```python
from build123d import *

# Parameters (mm, degrees)
F0_R     = 28.575
F0_R_2   = 2.032
F1_DEPTH = 3.175
F2_R     = 13.97
F3_DEPTH = 6.35
F5_DEPTH = 9.525
F7_DEPTH = 9.525
F8_R     = 12.954
F8_R_2   = 1.8288
F9_DEPTH = 3.175


with BuildPart() as f1:
    # F0 (on Top) → F1 (new body)
    with BuildSketch(Plane.XY):
        Circle(F0_R)
        with Locations((-20.6222299276, -11.90625)):
            Circle(F0_R_2, mode=Mode.SUBTRACT)
        with Locations((0, -23.8125)):
            Circle(F0_R_2, mode=Mode.SUBTRACT)
        with Locations((20.6222299276, -11.90625)):
            Circle(F0_R_2, mode=Mode.SUBTRACT)
        with Locations((-20.6222299276, 11.90625)):
            Circle(F0_R_2, mode=Mode.SUBTRACT)
        with Locations((20.6222299276, 11.90625)):
            Circle(F0_R_2, mode=Mode.SUBTRACT)
        with Locations((0, 23.8125)):
            Circle(F0_R_2, mode=Mode.SUBTRACT)
    extrude(amount=F1_DEPTH)

    # F2 (on face) → F3 (join)
    with BuildSketch(Plane.XY.offset(3.175)):
        Circle(F2_R)
    extrude(amount=F3_DEPTH)

    # F4 (on face) → F5 (cut, through all)
    with BuildSketch(Plane(origin=(0, 0, 0), x_dir=(1, 0, 0), z_dir=(0, 0, -1))):
        with BuildLine():
            ThreePointArc((-1.987864432, 2.794), (-1.5718864244, -3.0474930793), (3.429, 0))
            ThreePointArc((3.429, 0), (3.0474930793, 1.5718864244), (1.987864432, 2.794))
            Line((1.987864432, 2.794), (0, 2.794))
            Line((0, 2.794), (-1.987864432, 2.794))
        make_face()
    extrude(amount=-F5_DEPTH, mode=Mode.SUBTRACT)

    # F6 (on face) → F7 (cut, through all)
    with BuildSketch(Plane(origin=(0, 0, 0), x_dir=(1, 0, 0), z_dir=(0, 0, -1))):
        with BuildLine():
            Line((-6.9147972132, -6.9147972132), (-5.0859972132, -6.9147972132))
            ThreePointArc((-5.0859972132, -6.9147972132), (-5.6216403318, -5.6216403318), (-6.9147972132, -5.0859972132))
            Line((-6.9147972132, -5.0859972132), (-6.9147972132, -6.9147972132))
        make_face()
        with BuildLine():
            ThreePointArc((-6.9147972132, -5.0859972132), (-8.2079540947, -8.2079540947), (-5.0859972132, -6.9147972132))
            Line((-5.0859972132, -6.9147972132), (-6.9147972132, -6.9147972132))
            Line((-6.9147972132, -6.9147972132), (-6.9147972132, -5.0859972132))
        make_face()
        with BuildLine():
            Line((-6.9147972132, 6.9147972132), (-6.9147972132, 5.0859972132))
            ThreePointArc((-6.9147972132, 5.0859972132), (-5.6216403318, 5.6216403318), (-5.0859972132, 6.9147972132))
            Line((-5.0859972132, 6.9147972132), (-6.9147972132, 6.9147972132))
        make_face()
        with BuildLine():
            ThreePointArc((-5.0859972132, 6.9147972132), (-8.2079540947, 8.2079540947), (-6.9147972132, 5.0859972132))
            Line((-6.9147972132, 5.0859972132), (-6.9147972132, 6.9147972132))
            Line((-6.9147972132, 6.9147972132), (-5.0859972132, 6.9147972132))
        make_face()
        with BuildLine():
            Line((6.9147972132, 6.9147972132), (6.9147972132, 5.0859972132))
            ThreePointArc((6.9147972132, 5.0859972132), (8.2079540947, 5.6216403318), (8.7435972132, 6.9147972132))
            ThreePointArc((8.7435972132, 6.9147972132), (6.9147972132, 8.7435972132), (5.0859972132, 6.9147972132))
            Line((5.0859972132, 6.9147972132), (6.9147972132, 6.9147972132))
        make_face()
        with BuildLine():
            ThreePointArc((5.0859972132, 6.9147972132), (5.6216403318, 5.6216403318), (6.9147972132, 5.0859972132))
            Line((6.9147972132, 5.0859972132), (6.9147972132, 6.9147972132))
            Line((6.9147972132, 6.9147972132), (5.0859972132, 6.9147972132))
        make_face()
        with BuildLine():
            ThreePointArc((6.9147972132, -5.0859972132), (5.6216403318, -5.6216403318), (5.0859972132, -6.9147972132))
            Line((5.0859972132, -6.9147972132), (6.9147972132, -6.9147972132))
            Line((6.9147972132, -6.9147972132), (6.9147972132, -5.0859972132))
        make_face()
        with BuildLine():
            Line((6.9147972132, -6.9147972132), (5.0859972132, -6.9147972132))
            ThreePointArc((5.0859972132, -6.9147972132), (6.9147972132, -8.7435972132), (8.7435972132, -6.9147972132))
            ThreePointArc((8.7435972132, -6.9147972132), (8.2079540947, -5.6216403318), (6.9147972132, -5.0859972132))
            Line((6.9147972132, -5.0859972132), (6.9147972132, -6.9147972132))
        make_face()
    extrude(amount=-F7_DEPTH, mode=Mode.SUBTRACT)

    # F8 (on face) → F9 (cut)
    with BuildSketch(Plane.XY.offset(9.525)):
        Circle(F8_R)
        with Locations((-6.9147972132, -6.9147972132)):
            Circle(F8_R_2, mode=Mode.SUBTRACT)
        with Locations((6.9147972132, -6.9147972132)):
            Circle(F8_R_2, mode=Mode.SUBTRACT)
        with BuildLine():
            ThreePointArc((-1.987864432, -2.794), (0, 3.429), (1.987864432, -2.794))
            Line((1.987864432, -2.794), (-1.987864432, -2.794))
        make_face(mode=Mode.SUBTRACT)
        with Locations((-6.9147972132, 6.9147972132)):
            Circle(F8_R_2, mode=Mode.SUBTRACT)
        with Locations((6.9147972132, 6.9147972132)):
            Circle(F8_R_2, mode=Mode.SUBTRACT)
    extrude(amount=-F9_DEPTH, mode=Mode.SUBTRACT)


solid = f1.part
```
Work out the finished part from the listing and answer in its coordinate system (mm). A direction names the side the tool comes from. Coordinates: 2 decimals unless noted, no trailing zeros. Write each loop counter-clockwise with the first axis right and the second up, starting at its lowest first coordinate (ties: lowest second). Pieces come first, ordered by that corner, then holes.
Q1. Which of the six approach directions +Z, -Z, +X, -X, +Y, -Y give full straight-line access (tool end or side, diameter ignored) to faces 5 (the face through (6, 13, 3.175)), 6 (the face through (8.2, -10.3, 9.525)), 7 (the face through (0, -2.794, 3))?
Q2. Each of these flat-tipped pins is pushed along its axis until it touches: pin 1 Ø3 at (x, z) = (-1, 4.5) entering from +Y; pin 2 Ø6 at (x, y) = (-16, 14) entering from +Z (3 decimals); pin 3 Ø5 at (x, z) = (1.5, 7.5) entering from -Y. Where does it stop, or does it pass through?
Q3. Find the intervals of material crossed by line 1 (Y direction, x = 0, z = 2.1) (1 decimal); line 2 (Y direction, x = 0, z = 7.2); line 3 (Y direction, x = 7, z = 1.25), in increasing order.
Q4. A cutting plane is placed at A-A, the plane x = 0. State how many separate pieces and enclosed holes the cut face has, then the cut area to 3 significant figures.
Q5. Determine the mould class of faces 1 (the face through (-1.82, 13.85, 6.31)), 2 (the face through (21.715, 13.62, 1.565)), 3 (the face through (-22.652, -11.817, 1.565)), 4 (the face through (6, 0, 0)) for opening direction Y: released by +Y, released by -Y, zero draft, split by the parting line, or undercut.
Q6. A cutting plane is placed at B-B, the plane z = 5.25. Give the vertices of the cut face in (x, y), then the cut area to 3 significant figures.
Q7. A cutting plane is placed at D-D, the plane y = -20.5. Give the vertices of the cut face in (x, z) (3 decimals), then the cut area to 3 significant figures.
Findings below:
1. face 5: +Z
1. face 6: +Z, +X, -X, +Y, -Y
1. face 7: +Z, -Z
2. pin 1: stops at y = 28.57
2. pin 2: stops at z = 3.175
2. pin 3: stops at y = -13.97
3. line 1: y = -28.6 to -25.8, -21.8 to -2.8, 3.4 to 21.8, 25.8 to 28.6
3. line 2: y = -13.97 to -12.95, 12.95 to 13.97
3. line 3: y = -27.7 to -8.74, -5.09 to 5.09, 8.74 to 27.7
4. separate pieces: 4
4. enclosed holes: 0
4. area: 211 mm2
5. face 1: split by the parting line
5. face 2: undercut
5. face 3: undercut
5. face 4: zero draft
6. outline: circle Ø27.94 at (0, 0); hole circle Ø3.66 at (-6.91, -6.91); hole circle Ø3.66 at (-6.91, 6.91); hole (-1.99, -2.79) - (1.99, -2.79) arc R3.43 ccw (long way) to start; hole circle Ø3.66 at (6.91, -6.91); hole circle Ø3.66 at (6.91, 6.91)
6. area: 536 mm2
7. outline: (-19.907, 0) - (19.907, 0) - (19.907, 3.175) - (-19.907, 3.175) - close
7. area: 126 mm2
